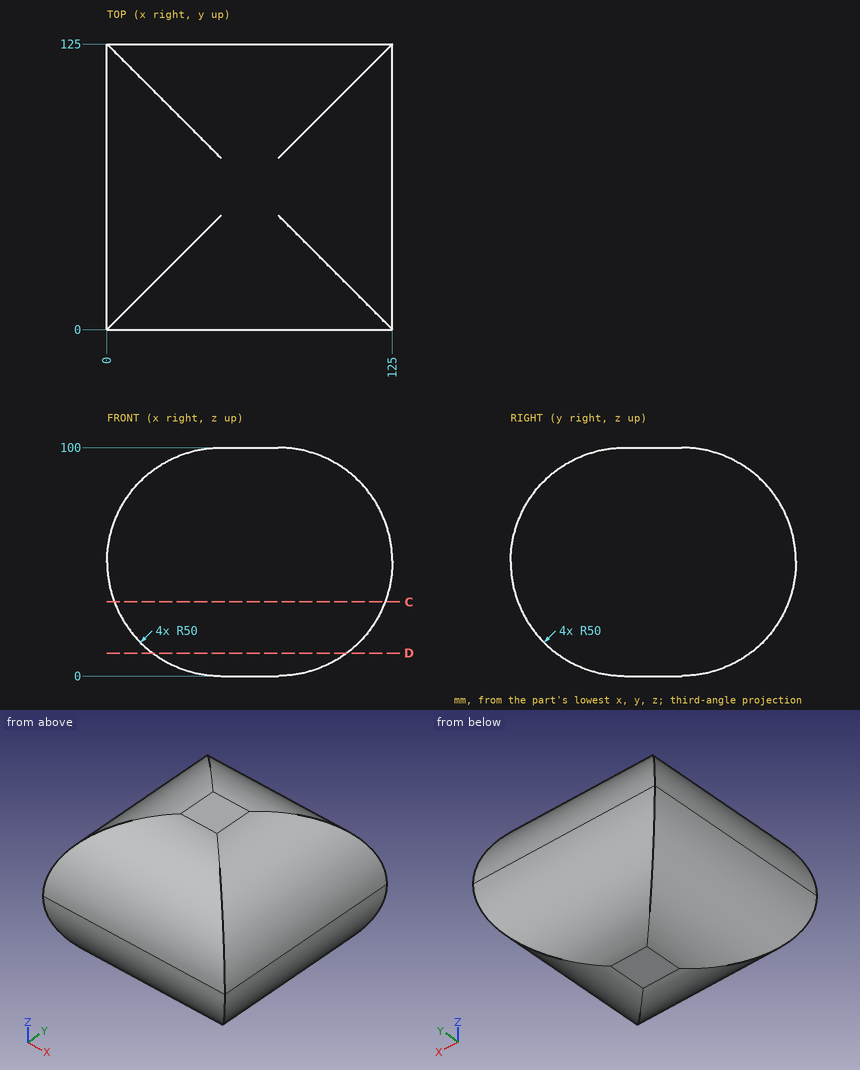
Answer from the drawing. Dimensions are ordinates in mm from the lowest x, y and z of the part. Round coordinates to 2 decimals unless told otherwise and drop trailing zeros. Loops run counter-clockwise (first coordinate to the right, second up) from the corner with the lowest first, then second, coordinate; pieces in that order, holes last. Notation, with made-up numbers: (18.25, -0.5) - (77.25, -0.5) arc R28 cw to (77.25, 21.5) - close; hole circle Ø11 at (4, 38). An arc over 180 degrees is marked (long way). Return JSON: item names as keys, results as strings. Group by question number.
1. Consider probe 1 along Y at (x, z) = (64, 50.5); probe 2 along X at (y, z) = (67.5, 48.5); probe 3 along Y at (x, z) = (80, 26). Determine where each line is inside the solid, lowest interval first.
2. Each of these flat-tipped pins is pushed along its axis until it touches: P1, Ø10, axis at y = 74.5, z = 65, coming from the -X side; P2, Ø1.5, axis at x = 107.5, y = 95, coming from the -Z side; P3, Ø4, axis at y = 94, z = 70, coming from the -X side. Where does it stop, or does it pass through?
3. The part is cut by section D-D on z = 10. Determine the outline of the cut face in (x, y), then the cut area to 4 significant figures.
4. The part is cut by section C-C on z = 32.5. Determine the outline of the cut face in (x, y), then the cut area to 3 significant figures.
Resolved:
{
 "1": {"probe 1": "y = 0 to 125", "probe 2": "x = 0.02 to 124.98", "probe 3": "y = 6.14 to 118.86"},
 "2": {"P1": "stops at x = 1.01", "P2": "stops at z = 11.37", "P3": "stops at x = 3.35"},
 "3": {"outline": "(20, 20) - (105, 20) - (105, 105) - (20, 105) - close", "area": "7,225 mm²"},
 "4": {"outline": "(3.16, 3.16) - (121.84, 3.16) - (121.84, 121.84) - (3.16, 121.84) - close", "area": "14,100 mm²"}
}
